Read the model definition and answer for the solid it produces. Units are mm, in the model's axes. Give positions to 0.01 mm unless a question says otherwise; leave off trailing zeros. Answer as CSV lines item,"result". Start each with the question number.
from build123d import *

# Parameters (mm, degrees)
SKETCH_1_W             = 508.938009882
SKETCH_1_H             = 8
EXTRUDE_1_DEPTH        = 30
EXTRUDE_2_DEPTH        = 30
PATTERN_LINEAR_1_COUNT = 54
PATTERN_LINEAR_1_PITCH = 9.424777961


with BuildPart() as part:
    # 草图1 → 拉伸1 (new body)
    with BuildSketch(Plane.XY):
        with Locations((254.469004941, -4)):
            Rectangle(SKETCH_1_W, SKETCH_1_H)
    extrude(amount=EXTRUDE_1_DEPTH)

    # 草图2 → 拉伸2 (add)
    with BuildSketch(Plane.XY.offset(30)):
        Polygon((0, 0), (2.456799081, 6.75), (4.985366656, 6.75), (7.442165737, 0), align=None)
    extrude_2 = extrude(amount=-EXTRUDE_2_DEPTH)

    # 阵列(线性)1: 拉伸2 ×54
    with Locations(*[(i * PATTERN_LINEAR_1_PITCH, 0, 0) for i in range(1, PATTERN_LINEAR_1_COUNT)]):
        add(extrude_2)


solid = part.part
(1) Flat-ended cylindrical pins translate along their axes: pin 1 Ø0.6 at (x, z) = (46.5, 14.5) entering from +Y; pin 2 Ø5 at (y, z) = (3, 3.5) entering from -X. Find the tip coordinate at first contact, or state that the pin passes through.
(2) Section A-A, the plane y = 4.5 is taken. State how many separate pieces and enclosed holes the cut face has, and give its area (3 significant figures).
(3) A straight line is drawn through the part: line 1 (Y direction, x = 65.5, z = 17). Find the intervals that lie inside material, in ascending order. Write a range as [from, to].
Checks:
1,pin 1,"stops at y = 0"
1,pin 2,"stops at x = 0.18"
2,separate pieces,"54"
2,enclosed holes,"0"
2,area,"6,750 mm²"
3,line 1,"y = [-8, 0]"
